Source: CAD feature listing. Evaluate the final solid. Frame: model axes, mm. A direction names the side the tool comes from. Give positions to 0.01 mm unless a question says otherwise; leave off trailing zeros. Write each loop counter-clockwise with the first axis right and the second up, starting at its lowest first coordinate (ties: lowest second). Pieces come first, ordered by that corner, then holes. Notation, with made-up numbers: (18.5, 69.5) -> (37.5, 69.5) arc R10 ccw to (37.5, 79.5) -> close; hole circle Ø4 at (72.25, 56). An arc over 180 degrees is marked (long way). Use one line per item in the form item = value. Start each with the question number.
(1) Cut plane A-A, the plane y = 86. Output: boundary loops of the cut face in (x, z).
(2) First-contact query: P1, Ø3, axis at y = -17.5, z = -1.5, coming from the +X side; P2, Ø4, axis at x = -1, y = -14.5, coming from the +Z side. Flat tips, straight axial feed; report the tip coordinate or a pass-through.
(3) Cut plane B-B, the plane y = 30.5. Output: boundary loops of the cut face in (x, z), and give its area (3 significant figures).
(4) Draft query along Y for faces 4 (the face through (6, 17, 0)), 5 (the face through (-2, -28, 2)), 6 (the face through (0, 60, -10.5)). Return one class per face: pulls with the +Y half, pulls with the -Y half, needs draft (parallel to the pull), parting line crosses it, or undercut.
(5) Set-up query: faces 1 (the face through (5.31, 29.9, -8.29)), 2 (the face through (-0.1, -29, -2.5)), 3 (the face through (-6, 17, 0)). Return all of +Z, -Z, +X, -X, +Y, -Y with unobstructed straight access to the full face (end or side cutting, diameter ignored); none if empty.
(6) Material intervals for line 1 along Y through (x, z) = (-6, 3.75); line 2 along Y through (x, z) = (-2.25, -7); line 3 along Y through (x, z) = (-2, 4.25), sorted ascending. Write a range as from..to.
from build123d import *

# Parameters (mm, degrees)
SKETCH_1_W            = 21
SKETCH_1_H            = 21
EXTRUDE_279_DEPTH     = 22.5
HOLE_WIZARD_4_0_4_1_D = 4
SKETCH_9_R            = 2.5
EXTRUDE_1_DEPTH       = 15
SKETCH_10_W           = 21
SKETCH_10_H           = 21
EXTRUDE_2_DEPTH       = 45


with BuildPart() as part:
    # Эскиз1 → Extrude 279 (new body)
    with BuildSketch(Plane(origin=(0, 0, 0), x_dir=(1, 0, 0), z_dir=(0, 1, 0))):
        Rectangle(SKETCH_1_W, SKETCH_1_H)
    extrude(amount=EXTRUDE_279_DEPTH)

    # Эскиз2 → Повернуть1 (revolve)
    with BuildSketch(Plane.XY, mode=Mode.PRIVATE) as revolve_1_sk:
        Polygon((0, 0), (6.5, 0), (6.5, -24.5), (3, -28), (0, -28), align=None)
    revolve(revolve_1_sk.sketch.rotate(Axis((0, -28, 0), (0, 1, 0)), 90), axis=Axis((0, -28, 0), (0, 1, 0)))

    # Диаметр отверстия Ø4.0 (4)1 (through all)
    with Locations(Plane.XY.offset(10.5)):
        with Locations((-6, 15), (6, 15)):
            Hole(HOLE_WIZARD_4_0_4_1_D / 2)

    # Эскиз8 → Повернуть4 (revolve)
    with BuildSketch(Plane.XY, mode=Mode.PRIVATE) as revolve_4_sk:
        Polygon((0.25, -28), (2.5, -28), (2.5, -30), (0.5, -48), (0.25, -48), align=None)
    revolve(revolve_4_sk.sketch.rotate(Axis((0, -28, 0), (0, -1, 0)), 90), axis=Axis((0, -28, 0), (0, -1, 0)))

    # Эскиз9 → Бобышка-Вытянуть1 (add)
    with BuildSketch(Plane(origin=(0, 22.5, 0), x_dir=(1, 0, 0), z_dir=(0, 1, 0))):
        with Locations(Location((-7.75, 7.75, 0), (0, 0, 270))):
            Circle(SKETCH_9_R)
        with Locations(Location((7.75, 7.75, 0), (0, 0, 270))):
            Circle(SKETCH_9_R)
        with Locations(Location((7.75, -7.75, 0), (0, 0, 270))):
            Circle(SKETCH_9_R)
        with Locations(Location((-7.75, -7.75, 0), (0, 0, 270))):
            Circle(SKETCH_9_R)
    extrude(amount=EXTRUDE_1_DEPTH)

    # Эскиз10 → Бобышка-Вытянуть2 (add)
    with BuildSketch(Plane(origin=(0, 37.5, 0), x_dir=(1, 0, 0), z_dir=(0, 1, 0))):
        Rectangle(SKETCH_10_W, SKETCH_10_H)
    extrude(amount=EXTRUDE_2_DEPTH)

    # Эскиз7 → Повернуть3 (revolve)
    with BuildSketch(Plane.XY, mode=Mode.PRIVATE) as revolve_3_sk:
        Polygon((0, 82.5), (0, 102.5), (9, 102.5), (9, 92.5), (3, 92.5), (3, 82.5), align=None)
    revolve(revolve_3_sk.sketch.rotate(Axis((0, 82.5, 0), (0, 1, 0)), 90), axis=Axis((0, 82.5, 0), (0, 1, 0)))


solid = part.part
Geometry says:
q1.outline = circle Ø6 at (0, 0)
q2.P1 = 6.5
q2.P2 = 6.5
q3.outline = circle Ø5 at (-7.75, -7.75); circle Ø5 at (-7.75, 7.75); circle Ø5 at (7.75, -7.75); circle Ø5 at (7.75, 7.75)
q3.area = 78.5 mm^2
q4.face_4 = undercut
q4.face_5 = pulls with the -Y half
q4.face_6 = needs draft
q5.face_1 = none
q5.face_2 = -Y
q5.face_3 = +Z, -Z
q6.line_1 = 0..13, 17..22.5, 37.5..82.5, 92.5..102.5
q6.line_2 = 0..22.5, 37.5..82.5, 92.5..102.5
q6.line_3 = -26.3..22.5, 37.5..82.5, 92.5..102.5
